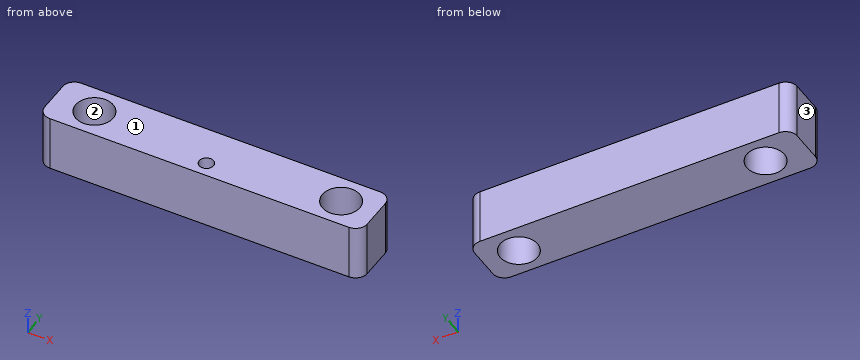
```python
from build123d import *

# Parameters (mm, degrees)
SKETCH5_W            = 175.006
SKETCH5_H            = 29.972
SKETCH5_R            = 10.16
BOSS_EXTRUDE11_DEPTH = 30.48
SKETCH7_R            = 3.887338421
CUT_EXTRUDE6_DEPTH   = 7.62
FILLET1_R            = 6.35


with BuildPart() as part:
    # Sketch5 → Boss-Extrude11 (new body)
    with BuildSketch(Plane.XY):
        with Locations((-72.157166667, 4.66725)):
            Rectangle(SKETCH5_W, SKETCH5_H)
        with Locations((-137.583333333, 4.66725)):
            Circle(SKETCH5_R, mode=Mode.SUBTRACT)
        with Locations((-3.715568727, 4.66725)):
            Circle(SKETCH5_R, mode=Mode.SUBTRACT)
    extrude(amount=BOSS_EXTRUDE11_DEPTH)

    # Sketch7 → Cut-Extrude6 (cut)
    with BuildSketch(Plane.XY.offset(30.48)):
        with Locations((-72.793003422, -2.423465595)):
            Circle(SKETCH7_R)
    extrude(amount=-CUT_EXTRUDE6_DEPTH, mode=Mode.SUBTRACT)

    # Fillet1
    fillet1_edges = [part.edges().sort_by_distance(p)[0] for p in [
        (15.345833333, -10.31875, 15.24),
        (-159.660166667, -10.31875, 15.24),
        (-159.660166667, 19.65325, 15.24),
        (15.345833333, 19.65325, 15.24),
    ]]
    fillet(fillet1_edges, radius=FILLET1_R)


solid = part.part
```
Build history of the part. All positions in model axes, mm. Face numbers are marked on the shaded views. Coordinates: 2 decimals unless noted, no trailing zeros. Order: outer loops, then holes, each group sorted by start corner. A loop starts at its lowest first (then second) coordinate and runs counter-clockwise, first axis right, second up. Notation, with made-up numbers: (45, -10.75) -> (69, -10.75) arc R15 ccw to (69, 11.25) -> close; hole circle Ø2 at (-38, 45.5). An arc over 180 degrees is marked (long way). Answer in a Markdown table with one row per item. Add a question column.
Q1. Drop flat-ended pins along their axis: pin 1 (6 mm diameter, centred on x = -72.79, y = -2.42, fed in from +Z); pin 2 (4 mm diameter, centred on y = -6.5, z = 25, fed in from +X); pin 3 (2 mm diameter, centred on x = -135.5, y = 13, fed in from -Z). Give the stop position or say it passes through.
Q2. Band-saw the part on A-A, the plane x = -6.5. List the corners of the cut face in (y, z), then the cut area to 3 significant figures.
Q3. Mould opens along X. For the marked faces 1, 2 and 3 say: +X half, -X half, draft (parallel to the pull), parting line (faces both ways), or undercut.
Q4. Band-saw the part on D-D, the plane z = 5. List the corners of the cut face in (x, y).
Q5. Band-saw the part on B-B, the plane z = 27. List the corners of the cut face in (x, y).
Q6. Band-saw the part on C-C, the plane y = 11.75. List the corners of the cut face in (x, z), then the cut area to 3 significant figures.
Q7. Wall check: line 1 along X through (y, z) = (1.5, 1); line 2 along X through (y, z) = (-3.5, 22.5); line 3 along Y through (x, z) = (-133.5, 1). Give the ranges that are in metal, low to high. Write a range as [from, to].
Answers follow:
| question | item | result |
|---|---|---|
| 1 | pin 1 | z = 22.86 |
| 1 | pin 2 | x = 15.32 |
| 1 | pin 3 | through |
| 2 | outline | (-10.32, 0) -> (-5.1, 0) -> (-5.1, 30.48) -> (-10.32, 30.48) -> close; (14.44, 0) -> (19.65, 0) -> (19.65, 30.48) -> (14.44, 30.48) -> close |
| 2 | area | 318 mm^2 |
| 3 | face 1 | draft |
| 3 | face 2 | undercut |
| 3 | face 3 | -X half |
| 4 | outline | (-159.66, -3.97) arc R6.35 ccw to (-153.31, -10.32) -> (9, -10.32) arc R6.35 ccw to (15.35, -3.97) -> (15.35, 13.3) arc R6.35 ccw to (9, 19.65) -> (-153.31, 19.65) arc R6.35 ccw to (-159.66, 13.3) -> close; hole circle Ø20.32 at (-137.58, 4.67); hole circle Ø20.32 at (-3.72, 4.67) |
| 5 | outline | (-159.66, -3.97) arc R6.35 ccw to (-153.31, -10.32) -> (9, -10.32) arc R6.35 ccw to (15.35, -3.97) -> (15.35, 13.3) arc R6.35 ccw to (9, 19.65) -> (-153.31, 19.65) arc R6.35 ccw to (-159.66, 13.3) -> close; hole circle Ø20.32 at (-137.58, 4.67); hole circle Ø7.77 at (-72.79, -2.42); hole circle Ø20.32 at (-3.72, 4.67) |
| 6 | outline | (-159.66, 0) -> (-144.87, 0) -> (-144.87, 30.48) -> (-159.66, 30.48) -> close; (-130.3, 0) -> (-11, 0) -> (-11, 30.48) -> (-130.3, 30.48) -> close; (3.57, 0) -> (15.35, 0) -> (15.35, 30.48) -> (3.57, 30.48) -> close |
| 6 | area | 4,450 mm^2 |
| 7 | line 1 | [-159.66, -147.24], [-127.93, -13.37], [5.94, 15.35] |
| 7 | line 2 | [-159.66, -143.63], [-131.54, -9.76], [2.33, 15.35] |
| 7 | line 3 | [-10.32, -4.64], [13.97, 19.65] |
